Autodesk Inventor part; units mm, degrees
ref_plane "YZ Plane" through (0, 0, 0) normal (1, 0, 0) x (0, 1, 0)
ref_plane "XZ Plane" through (0, 0, 0) normal (0, 1, 0) x (-1, 0, 0)
ref_plane "XY Plane" through (0, 0, 0) normal (0, 0, 1) x (1, 0, 0)
sketch "스케치13" plane through (0, 0, 0) normal (0, 0, 1) x (1, 0, 0)
  circle A0 centre (0, 0) radius 35
  dimension "d74" = 70
extrude "돌출11" add sketch "스케치13" along normal blind 7
sketch "스케치19" plane through (0, 0, 7) normal (0, 0, 1) x (1, 0, 0)
  circle A0 centre (0, 0) radius 20
  dimension "d92" = 40
extrude "돌출17" add sketch "스케치19" along normal blind 3
sketch "스케치20" plane through (0, 0, 10) normal (0, 0, 1) x (1, 0, 0)
  circle A0 centre (0, 0) radius 16
  dimension "d95" = 32
extrude "돌출18" cut sketch "스케치20" against normal blind 5
sketch "스케치16" plane through (0, 0, 0) normal (0, 0, -1) x (-1, 0, 0)
  circle A0 centre (0, 0) radius 23.5
  dimension "d83" = 47
extrude "돌출15" cut sketch "스케치16" against normal blind 3
sketch "스케치18" plane through (0, 0, 3) normal (0, 0, -1) x (-1, 0, 0)
  circle A0 centre (0, 0) radius 10.5
  dimension "d89" = 21
extrude "돌출16" cut sketch "스케치18" against normal up to next
fillet "모깎기3" radius 3 2 edges at (-20, 0, 10) (23.5, 0, 3)
sketch "스케치21" plane through (0, 0, 7) normal (0, 0, 1) x (1, 0, 0)
  circle A0 centre (0, 28) radius 4
  line L0 (-4, 28) -> (4, 28)
  line L1 (4, 28) -> (4, 38)
  line L2 (4, 38) -> (-4, 38)
  line L3 (-4, 38) -> (-4, 28)
  point P0 (0, 0)
  dimension "d99" = 8
  dimension "d100" = 28
extrude "돌출19" cut sketch "스케치21" against normal blind 4.4
sketch "스케치22" plane through (0, 0, 2.6) normal (0, 0, 1) x (1, 0, 0)
  arc A0 (-4, 28) -> (4, 28) centre (0, 28) ccw
  circle A1 centre (0, 28) radius 4
  point P0 (0, 0)
hole "구멍2" at (0, 28, 2.6) direction (0, 0, -1) diameter 4.5 end through all
pattern_circular "원형 패턴3" count 6 over 360 about axis through (0, 0, 3) along (0, 0, 1) of "돌출19", "구멍2"
properties part number "도면3-2번"
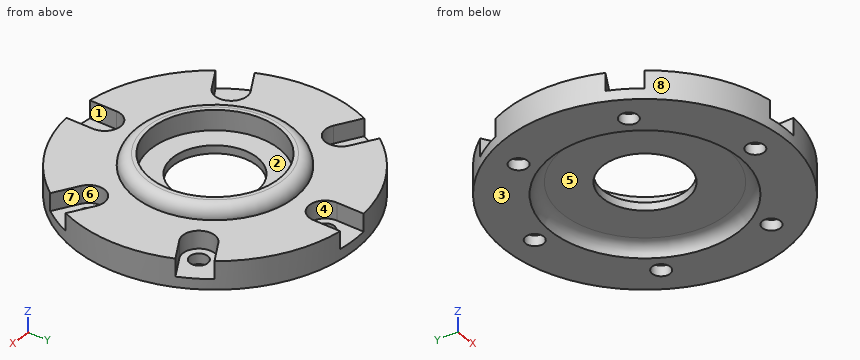
Geometry check sheet. Reference: the model listing, model coordinates, mm. Face numbers are marked on the shaded views. A direction names the side the tool comes from. Round coordinates to 2 decimals unless told otherwise and drop trailing zeros. Order: outer loops, then holes, each group sorted by start corner. A loop starts at its lowest first (then second) coordinate and runs counter-clockwise, first axis right, second up. Notation, with made-up numbers: M -11.5,-25 L 28.5,-25 A17 ccw 28.5,2 Z; hole C 35,46.25 d8. An arc over 180 degrees is marked long. Write item = value, one per line.
Q1. Scan lines: line 1 (X direction, y = 11.5, z = 4.75); line 2 (Z direction, x = 25, y = 5.5); line 3 (X direction, y = -28, z = 1.1). Record each from-to range of solid material in increasing order.
Answer block:
line_1 = -33.06 to -27.92, -21.13 to 21.13, 27.92 to 33.06
line_2 = 0 to 7
line_3 = -21 to -2.25, 2.25 to 21
Q2. Depth check by flat-ended pin: pin 1 Ø2 at (y, z) = (30, 5) entering from +X; pin 2 Ø6 at (x, y) = (0, 28) entering from -Z; pin 3 Ø7 at (x, y) = (24.25, -14) entering from +Z; pin 4 Ø1.5 at (x, y) = (8.5, 19.5) entering from -Z. Enter the tip coordinate at first touch or a pass-through.
Answer block:
pin_1 = 19.6
pin_2 = 0
pin_3 = 2.6
pin_4 = 2.59
Q3. Section check B-B (x = 0). Give the number of separate pieces and of enclosed holes in the cut face, plus the area to 3 significant figures.
Answer block:
separate_pieces = 4
enclosed_holes = 0
area = 147 mm^2
Q4. Set-up check for the marked faces 1, 2, 3, 4 and 5: record each of +Z, -Z, +X, -X, +Y, -Y from which the full face is reachable in a straight line by a thin tool's end or side.
Answer block:
face_1 = +Z, -Y
face_2 = +Z
face_3 = -Z, +X, -X, +Y, -Y
face_4 = +Z, +Y
face_5 = -Z
Q5. Release check for a two-part mould opening along X. For the marked faces 6, 7 and 8 record: released by +X, released by -X, zero draft, split by the parting line, or undercut.
Answer block:
face_6 = undercut
face_7 = released by +X
face_8 = split by the parting line
Q6. Section check A-A (z = 1.75). Enter the section's corners in (x, y) (3 decimals).
Answer block:
outline = C 0,0 d70; hole C -24.249,-14 d4.5; hole C -24.249,14 d4.5; hole C 0,0 d45.874; hole C 0,-28 d4.5; hole C 0,28 d4.5; hole C 24.249,-14 d4.5; hole C 24.249,14 d4.5
